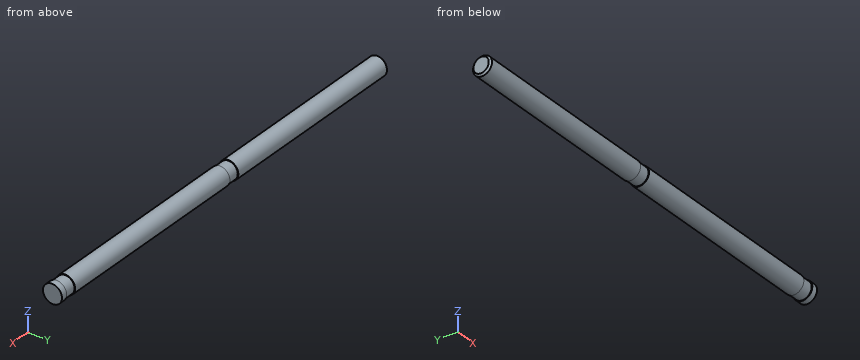
from build123d import *

# Parameters (mm, degrees)
F0_R     = 3.96875
F1_DEPTH = 176.276
F2_W     = 4.572
F2_H     = 1.702164
F4_SIZE2 = 0.762
F4_SIZE  = 0.762


with BuildPart() as f1:
    # F0 (on Right) → F1 (new body)
    with BuildSketch(Plane.YZ):
        Circle(F0_R)
    extrude(amount=F1_DEPTH)

    # F2 (on Front) → F3 (revolve, cut)
    with BuildSketch(Plane.XZ):
        with Locations((171.45, 4.572182)):
            Rectangle(F2_W, F2_H)
        with Locations((83.312, 4.572182)):
            Rectangle(F2_W, F2_H)
    revolve(axis=Axis((171.45, 0, 0), (-1, 0, 0)), mode=Mode.SUBTRACT)

    # F4
    f4_edges = [f1.edges().sort_by_distance(p)[0] for p in [
        (0, -3.96875, 0),
    ]]
    chamfer(f4_edges, length=F4_SIZE, length2=F4_SIZE2)


solid = f1.part
Input: part model. Units: mm. Frame: model coordinates. Coordinates: 2 decimals unless noted, no trailing zeros. Loops run counter-clockwise (first coordinate to the right, second up) from the corner with the lowest first, then second, coordinate; pieces in that order, holes last.
Q1. Material intervals for line 1 (X direction, y = -3.5, z = -1.75); line 2 (X direction, y = 2.25, z = -3); line 3 (Z direction, x = 139.5, y = -0.5), sorted ascending.
Q2. Cut plane A-A (x = 119). Output: boundary loops of the cut face in (y, z), then the cut area to 3 significant figures.
Q3. Contact query for flat-ended pins moving along their axis: pin 1 (2.5 mm diameter, centred on y = 0.5, z = 0, fed in from -X); pin 2 (2 mm diameter, centred on x = 22, z = -3, fed in from -Y); pin 3 (4 mm diameter, centred on x = 131.5, z = 2.5, fed in from -Y). Output: stop coordinate, or through.
Working result:
1. line 1: x = 0.71 to 81.03, 85.6 to 169.16, 173.74 to 176.28
1. line 2: x = 0.54 to 81.03, 85.6 to 169.16, 173.74 to 176.28
1. line 3: z = -3.94 to 3.94
2. outline: circle Ø7.94 at (0, 0)
2. area: 49.5 mm2
3. pin 1: stops at x = 0
3. pin 2: stops at y = -3.43
3. pin 3: stops at y = -3.94
